Autodesk Inventor part; units mm, degrees
ref_plane "YZ Plane" through (0, 0, 0) normal (1, 0, 0) x (0, 1, 0)
ref_plane "XZ Plane" through (0, 0, 0) normal (0, 1, 0) x (-1, 0, 0)
ref_plane "XY Plane" through (0, 0, 0) normal (0, 0, 1) x (1, 0, 0)
sketch "Skizze1" plane through (0, 0, 0) normal (0, 0, 1) x (1, 0, 0)
  line L0 (0, 0) -> (50, 0)
  line L1 (50, 0) -> (50, 50)
  line L2 (50, 50) -> (0, 50)
  line L3 (0, 50) -> (0, 0)
  dimension "d0" = 50
  dimension "d1" = 50
extrude "Extrusion1" add sketch "Skizze1" along normal blind 2
sketch "Skizze3" plane through (0, 0, 2) normal (0, 0, 1) x (1, 0, 0)
  line L0 (0, 0) -> (0, 50)
  line L1 (50, 0) -> (0, 0)
  line L2 (50, 50) -> (50, 0)
  line L3 (0, 50) -> (50, 50)
  line L4 (2, 48) -> (2, 2)
  line L5 (2, 2) -> (48, 2)
  line L6 (48, 2) -> (48, 48)
  line L7 (48, 48) -> (2, 48)
  dimension "d15" = 2
hole "Bohrung2" at (2, 48, 2) at (48, 48, 2) at (48, 2, 2) at (2, 2, 2) direction (0, 0, -1) diameter 2.4 end through all
properties part number "1_0204_004"
Geometry: final body of the model. Coordinates: model frame, mm. Round coordinates to 2 decimals unless told otherwise and drop trailing zeros. Order: outer loops, then holes, each group sorted by start corner. A loop starts at its lowest first (then second) coordinate and runs counter-clockwise, first axis right, second up.
Q1. Mould query, pull axis Y, two halves, no side actions, for faces 1 (the face through (2.46, 46.89, 0.99)), 2 (the face through (25, 50, 1)), 3 (the face through (25, 0, 1)), 4 (the face through (47.64, 46.855, 0.986)). Classes: released by +Y, released by -Y, zero draft, split by the parting line, or undercut.
Result sheet:
face 1: undercut
face 2: released by +Y
face 3: released by -Y
face 4: undercut
Q2. Pin query (flat end, axial travel): pin 1 (2 mm diameter, centred on x = 2, y = 48, fed in from +Z). Return the tip coordinate at first contact, or that it passes through.
Result sheet:
pin 1: passes through
Q3. Section A-A, the plane y = 2. Output: boundary loops of the cut face in (x, z), and give its area (3 significant figures).
Result sheet:
outline: (0, 0) - (0.8, 0) - (0.8, 2) - (0, 2) - close; (3.2, 0) - (46.8, 0) - (46.8, 2) - (3.2, 2) - close; (49.2, 0) - (50, 0) - (50, 2) - (49.2, 2) - close
area: 90.4 mm2
Q4. Material intervals for probe 1 along Y at (x, z) = (48, 1.45); probe 2 along X at (y, z) = (47.5, 1.9), sorted ascending.
Result sheet:
probe 1: y = 0 to 0.8, 3.2 to 46.8, 49.2 to 50
probe 2: x = 0 to 0.91, 3.09 to 46.91, 49.09 to 50
